Autodesk Inventor part; units mm, degrees
ref_plane "YZ Plane" through (0, 0, 0) normal (1, 0, 0) x (0, 1, 0)
ref_plane "XZ Plane" through (0, 0, 0) normal (0, 1, 0) x (-1, 0, 0)
ref_plane "XY Plane" through (0, 0, 0) normal (0, 0, 1) x (1, 0, 0)
sketch "Sketch1" plane through (0, 0, 0) normal (0, 1, 0) x (-1, 0, 0)
  line L0 (0, 0) -> (0, -39.8)
  line L1 (0, -39.8) -> (55.8, -39.8)
  line L2 (55.8, -39.8) -> (55.8, 0)
  line L3 (55.8, 0) -> (0, 0)
  line L4 (7.8, -7.8) -> (7.8, -32)
  line L5 (7.8, -32) -> (48, -32)
  line L6 (48, -32) -> (48, -7.8)
  line L7 (48, -7.8) -> (7.8, -7.8)
  line L8 (3.9, -3.9) -> (3.9, -35.9) construction
  line L9 (3.9, -35.9) -> (51.9, -35.9) construction
  line L10 (51.9, -35.9) -> (51.9, -3.9) construction
  line L11 (51.9, -3.9) -> (3.9, -3.9) construction
  circle A0 centre (3.9, -3.9) radius 1.5
  circle A1 centre (3.9, -35.9) radius 1.5
  circle A2 centre (51.9, -3.9) radius 1.5
  circle A3 centre (51.9, -35.9) radius 1.5
  circle A4 centre (3.9, -35.9) radius 3
  circle A5 centre (3.9, -3.9) radius 3
  circle A6 centre (51.9, -3.9) radius 3
  circle A7 centre (51.9, -35.9) radius 3
  dimension "d0" = 39.8
  dimension "d1" = 55.8
  dimension "d4" = 24.2
  dimension "d5" = 40.2
  dimension "d6" = 7.8
  dimension "d7" = 7.8
  dimension "d8" = 32
  dimension "d9" = 48
  dimension "d10" = 3.9
  dimension "d11" = 3.9
  dimension "d12" = 3
  dimension "d14" = 3
  dimension "d15" = 3
  dimension "d16" = 3
  dimension "d17" = 6
  dimension "d19" = 6
  dimension "d20" = 6
  dimension "d22" = 6
extrude "Extrusion1" add sketch "Sketch1" along normal blind 8 contours L3 L2 L1 L0
extrude "Extrusion13" add sketch "Sketch1" along normal blind 2 from surface at 8 separate body contours L3 L2 L1 L0
extrude "Extrusion12" add sketch "Sketch1" against normal blind 2 separate body contours L3 L2 L1 L0
extrude "Extrusion2" add sketch "Sketch1" along normal blind 2 from surface at -2 contours A4 | A5 | A6 | A7 bodies 1
extrude "Extrusion3" add sketch "Sketch1" against normal blind 6 from surface at -2 contours A4 | A5 | A6 | A7 bodies 1
sketch "Sketch2" plane through (0, 0, 0) normal (1, 0, 0) x (0, 0, -1)
  line L0 (0, 0) -> (0, 8) construction
  line L1 (0, 8) -> (39.8, 8) construction
  line L2 (39.8, 0) -> (39.8, 8) construction
  line L3 (0, 0) -> (39.8, 0) construction
  line L4 (0, 4) -> (39.8, 4) construction
  line L5 (19.9, 8) -> (19.9, 0) construction
  circle A0 centre (19.9, 4) radius 2.4
  dimension "d30" = 4.8
extrude "Extrusion4" cut sketch "Sketch2" against normal up to surface (7.8 mm away) bodies 1
sketch "Sketch3" plane through (0, 0, -39.8) normal (0, 0, -1) x (-1, 0, 0)
  line L0 (0, 8) -> (55.8, 8) construction
  line L1 (0, 0) -> (0, 8) construction
  line L2 (0, 0) -> (55.8, 0) construction
  line L3 (55.8, 0) -> (55.8, 8) construction
  line L4 (27.9, 8) -> (27.9, 0) construction
  line L5 (0, 4) -> (55.8, 4) construction
  circle A0 centre (11.9, 4) radius 4
  circle A1 centre (11.9, 4) radius 1.5
  circle A2 centre (43.9, 4) radius 4
  circle A3 centre (43.9, 4) radius 1.5
  line L6 (20.4, 0) -> (35.4, 0)
  line L7 (35.4, 0) -> (35.4, 8)
  line L8 (35.4, 8) -> (20.4, 8)
  line L9 (20.4, 8) -> (20.4, 0)
  line L10 (27.9, 8) -> (27.9, 0) construction
  line L11 (20.4, 4) -> (35.4, 4) construction
  line L12 (23.9, 8) -> (23.9, 0)
  line L13 (31.9, 0) -> (31.9, 8)
  point P0 (27.9, 4)
  dimension "d34" = 16
  dimension "d35" = 8
  dimension "d36" = 3
  dimension "d49" = 15
  dimension "d50" = 8
  dimension "d55" = 4
  dimension "d56" = 4
extrude "Extrusion10" cut sketch "Sketch3" against normal up to surface (7.8 mm away) contours L12 L8 L13 L6 bodies 1
extrude "Extrusion9" cut sketch "Sketch3" along normal blind 4 from surface at -7.8 contours L9 L8 L12 L6 | L13 L8 L7 L6 bodies 1
extrude "Extrusion6" add sketch "Sketch3" along normal blind 12.1 contours A0 | A2 bodies 1
sketch "Sketch4" plane through (-55.8, 0, 0) normal (0, 0, 1) x (1, 0, 0)
  line L0 (0, 8) -> (55.8, 8) construction
  line L1 (0, 0) -> (0, 8) construction
  line L2 (0, 0) -> (55.8, 0) construction
  line L3 (55.8, 0) -> (55.8, 8) construction
  line L4 (27.9, 8) -> (27.9, 0) construction
  line L5 (0, 4) -> (55.8, 4) construction
  circle A0 centre (11.9, 4) radius 4
  circle A1 centre (11.9, 4) radius 1.5
  circle A2 centre (43.9, 4) radius 4
  circle A3 centre (43.9, 4) radius 1.5
  line L6 (20.4, 0) -> (35.4, 0)
  line L7 (35.4, 0) -> (35.4, 8)
  line L8 (35.4, 8) -> (20.4, 8)
  line L9 (20.4, 8) -> (20.4, 0)
  line L10 (27.9, 8) -> (27.9, 0) construction
  line L11 (20.4, 4) -> (35.4, 4) construction
  line L12 (23.9, 8) -> (23.9, 0)
  line L13 (31.9, 0) -> (31.9, 8)
  line L14 (0, 8) -> (55.8, 8) construction
  line L15 (0, 0) -> (0, 8) construction
  line L16 (0, 0) -> (55.8, 0) construction
  line L17 (55.8, 0) -> (55.8, 8) construction
  point P0 (27.9, 4)
  dimension "d59" = 16
  dimension "d60" = 8
  dimension "d61" = 3
  dimension "d62" = 15
  dimension "d63" = 8
  dimension "d64" = 4
  dimension "d65" = 4
extrude "Extrusion7" cut sketch "Sketch4" against normal up to surface (7.8 mm away) contours L12 L8 L13 L6 bodies 1
extrude "Extrusion11" cut sketch "Sketch4" along normal blind 4 from surface at -7.8 contours L9 L8 L12 L6 | L13 L8 L7 L6 bodies 1
extrude "Extrusion8" add sketch "Sketch4" along normal blind 12.1 contours A0 | A2 bodies 1
combine bodies "Combine1" operation type add bodies to combine 1 3 2
equation "\"d7\" = d6"
equation "\"d10\" = 0.5 * d6"
equation "\"d11\" = 0.5 * d6"
equation "\"d12\" = d14"
equation "\"d15\" = d14"
equation "\"d16\" = d14"
equation "\"d19\" = d17"
equation "\"d20\" = d21"
equation "\"d22\" = d23"
equation "\"d55\" = 0.5 * d50"
equation "\"d56\" = 0.5 * d50"
equation "\"d64\" = 0.5 * d63"
equation "\"d65\" = 0.5 * d63"
properties part number "diff_gear_holder"
CAD build for the part. Positions are in the model's coordinates, mm. A direction names the side the tool comes from. Round coordinates to 2 decimals unless told otherwise and drop trailing zeros. Loops run counter-clockwise (first coordinate to the right, second up) from the corner with the lowest first, then second, coordinate; pieces in that order, holes last. Notation, with made-up numbers: (65, 58.25) - (99, 58.25) arc R24 ccw to (99, 73.25) - close; hole circle Ø3 at (-37, 34). An arc over 180 degrees is marked (long way). Return JSON: item names as keys, results as strings. Group by question number.
Q1. Two-plate mould, pull along Z, no slides. Class faces 5 (the face through (-45.33, 3.55, -45.77)), 6 (the face through (-44, 4, 0)), 7 (the face through (-53.33, -4.06, -4.35)): +Z half, -Z half, draft (parallel to the pull), parting line (faces both ways), or undercut.
Q2. Tool access for faces 1 (the face through (-45.1, 4.9, 6)), 2 (the face through (-28, 0, -35)), 3 (the face through (-5.2, 0, -37.2)), 4 (the face through (-23.9, 4, -2)): list every direction of +Z, -Z, +X, -X, +Y, -Y with a clear straight run to the whole face (end or side of a thin tool).
Q3. Drill centre lines: line 1 along Z through (x, y) = (-3.9, -4); line 2 along Z through (x, y) = (-36, 1.75); line 3 along Y through (x, z) = (-31.5, -4). Where is each one in solid material? Low to high. Write a range as [from, to].
Q4. Band-saw the part on B-B on x = -3.9. Give the number of separate pieces and of enclosed holes in the cut face, plus the area to 3 significant figures.
Q5. Band-saw the part on D-D on z = -16. Give the cut face in (x, y).
Q6. Band-saw the part on C-C on x = -51.9. Give the cut face in (y, z), plus the area to 3 significant figures.
Q7. Band-saw the part on A-A on y = -3.75. Give the cut face in (x, z), plus the area to 3 significant figures.
Q8. Flat gauge pins, fed straight in: pin 1 Ø2 at (x, z) = (-44, -3) entering from -Y; pin 2 Ø4.5 at (y, z) = (4, -19.9) entering from +X; pin 3 Ø3 at (x, z) = (-4.5, -35) entering from +Y; pin 4 Ø3.5 at (x, y) = (-11.9, 4) entering from -Z. Where does each tip first touch, or does it go through?
Solutions:
{
 "1": {"face 5": "draft", "face 6": "+Z half", "face 7": "undercut"},
 "2": {"face 1": "+Z", "face 2": "none", "face 3": "+Y", "face 4": "+Z, -Z"},
 "3": {"line 1": "z = [-38.9, -37.4], [-34.4, -32.9], [-6.9, -5.4], [-2.4, -0.9]", "line 2": "z = [-39.8, -32], [-7.8, 0]", "line 3": "y = [-2, 0], [8, 10]"},
 "4": {"separate pieces": "3", "enclosed holes": "1", "area": "364 mm^2"},
 "5": {"outline": "(-55.8, -2) - (-48, -2) - (-48, 10) - (-55.8, 10) - close; (-7.8, -2) - (0, -2) - (0, 10) - (-7.8, 10) - close"},
 "6": {"outline": "(-8, -38.9) - (-2, -38.9) - (-2, -39.8) - (10, -39.8) - (10, -38.9) - (0, -38.9) - (0, -37.4) - (-8, -37.4) - close; (-8, -34.4) - (0, -34.4) - (0, -32.9) - (10, -32.9) - (10, -6.9) - (0, -6.9) - (0, -5.4) - (-8, -5.4) - (-8, -6.9) - (-2, -6.9) - (-2, -32.9) - (-8, -32.9) - close; (-8, -2.4) - (0, -2.4) - (0, -0.9) - (10, -0.9) - (10, 0) - (-2, 0) - (-2, -0.9) - (-8, -0.9) - close", "area": "382 mm^2"},
 "7": {"outline": "circle Ø6 at (-51.9, -35.9); circle Ø6 at (-51.9, -3.9); circle Ø6 at (-3.9, -35.9); circle Ø6 at (-3.9, -3.9); hole circle Ø3 at (-51.9, -35.9); hole circle Ø3 at (-51.9, -3.9); hole circle Ø3 at (-3.9, -35.9); hole circle Ø3 at (-3.9, -3.9)", "area": "84.8 mm^2"},
 "8": {"pin 1": "stops at y = -2", "pin 2": "stops at x = -48", "pin 3": "stops at y = 0", "pin 4": "stops at z = -51.9"}
}
